CAD build for the part. Positions are in the model's coordinates, mm. A direction names the side the tool comes from. Round coordinates to 2 decimals unless told otherwise and drop trailing zeros. Loops run counter-clockwise (first coordinate to the right, second up) from the corner with the lowest first, then second, coordinate; pieces in that order, holes last. Notation, with made-up numbers: M 60.25,22.5 L 65.25,22.5 A23 ccw 65.25,44.5 Z; hole C 49,-3.75 d8. An arc over 180 degrees is marked long. Use a Markdown table: item, result. Add a question column.
(1) Wall check: L1, parallel to Z at x = 4.5, y = 1.2; L2, parallel to Z at x = 0, y = 0.6; L3, parallel to X at y = 0.6, z = -2.3. Give the ranges that are in metal, low to high.
(2) Band-saw the part on A-A, the plane z = -3.1. Write the cut outline in (x, y).
(3) Two-plate mould, pull along X, no slides. Class faces 4 (the face through (-0.37, 1.5, -3.64)), 5 (the face through (0.1, 0.7, -3.5)), 6 (the face through (-4.025, 0.944, -0.232)), 7 (the face through (0, 1, -4)): released by +X, released by -X, zero draft, split by the parting line, or undercut.
(4) Band-saw the part on C-C, the plane x = 0. Write the cut outline in (y, z).
(5) Band-saw the part on D-D, the plane z = -2.25. Write the cut outline in (x, y), and give its area (3 significant figures).
(6) Band-saw the part on B-B, the plane y = 0.1. Write the cut outline in (x, z).
(7) Which spindle directions (+Z, -Z, +X, -X, +Y, -Y) get a long thin tool onto all of the face, cutting with end or side? Do faces 1 (the face through (5, 1, -0.47)), 2 (the face through (-5.14, 0.74, -0.47)), 3 (the face through (4, 1, 0)). Say none if no direction does.
from build123d import *

# Parameters (mm, degrees)
BOSS_EXTRUDE1_DEPTH = 1.5
SKETCH3_R           = 0.482388485
CUT_EXTRUDE1_DEPTH  = 0.47


with BuildPart() as part:
    # Sketch1 → Boss-Extrude1 (new body)
    with BuildSketch(Plane(origin=(0, 0, 0), x_dir=(1, 0, 0), z_dir=(0, 1, 0))):
        with BuildLine():
            Line((5.365482369, 0), (3.5, 0))
            ThreePointArc((3.5, 0), (0, 3.5), (-3.5, 0))
            Line((-3.5, 0), (-5.365482369, 0))
            Line((-5.365482369, 0), (-5.365482369, 0.469939432))
            Line((-5.365482369, 0.469939432), (-3.972298696, 0.469939432))
            ThreePointArc((-3.972298696, 0.469939432), (0, 4), (3.972298696, 0.469939432))
            Line((3.972298696, 0.469939432), (5.365482369, 0.469939432))
            Line((5.365482369, 0.469939432), (5.365482369, 0))
        make_face()
    extrude(amount=BOSS_EXTRUDE1_DEPTH)

    # Sketch3 → Cut-Extrude1 (cut)
    with BuildSketch(Plane.XY):
        with Locations((-4.485222017, 0.798824848)):
            Circle(SKETCH3_R)
    extrude(amount=-CUT_EXTRUDE1_DEPTH, mode=Mode.SUBTRACT)


solid = part.part
Return value:
| question | item | result |
|---|---|---|
| 1 | L1 | -0.47 to 0 |
| 1 | L2 | -4 to -3.5 |
| 1 | L3 | -3.27 to -2.64, 2.64 to 3.27 |
| 2 | outline | M -2.53,0 L -1.62,0 L -1.62,1.5 L -2.53,1.5 Z; M 1.62,0 L 2.53,0 L 2.53,1.5 L 1.62,1.5 Z |
| 3 | face 4 | zero draft |
| 3 | face 5 | undercut |
| 3 | face 6 | undercut |
| 3 | face 7 | split by the parting line |
| 4 | outline | M 0,-4 L 1.5,-4 L 1.5,-3.5 L 0,-3.5 Z |
| 5 | outline | M -3.31,0 L -2.68,0 L -2.68,1.5 L -3.31,1.5 Z; M 2.68,0 L 3.31,0 L 3.31,1.5 L 2.68,1.5 Z |
| 5 | area | 1.88 mm^2 |
| 6 | outline | M -5.37,-0.47 L -3.97,-0.47 A4 ccw 3.97,-0.47 L 5.37,-0.47 L 5.37,0 L 3.5,0 A3.5 cw -3.5,0 L -5.37,0 Z |
| 7 | face 1 | -Z, +X, +Y, -Y |
| 7 | face 2 | -Z, -X, +Y, -Y |
| 7 | face 3 | +Z, +X, -X, +Y, -Y |
